Here's how the part is built. I have some questions about the finished solid (model axes, mm). Face numbers are marked on the shaded views. A direction names the side the tool comes from. Coordinates: 2 decimals unless noted, no trailing zeros. Write each loop counter-clockwise with the first axis right and the second up, starting at its lowest first coordinate (ties: lowest second). Pieces come first, ordered by that corner, then holes. Notation, with made-up numbers: (61, 14.5) - (118, 14.5) arc R27 ccw to (118, 50.5) - close; hole circle Ø8 at (-5, -39). An arc over 180 degrees is marked (long way). Answer in a Markdown table with one row per item. Add a question column.
Item 1: Which directions (+Z, -Z, +X, -X, +Y, -Y) give clear straight access to the entire face, cutting with the end or side of a thin tool? Please do the marked faces 1 and 2.
Item 2: Imagine slicing it at C-C (x = -13). Please give me the cut outline in (y, z), plus the area to 3 significant figures.
Item 3: I'm going to push a flat-ended pin straight in: pin 1 (10 mm diameter, centred on x = 4, y = -33, fed in from -Z). Where does the tip first touch, or does it pass through?
Item 4: If I drill on probe 1 along X at (y, z) = (-14.5, 38); probe 2 along Z at (x, y) = (-0.5, -12), over which ranges is the centre line in solid material (lowest first)? Write a range as from..to.
Item 5: Imagine slicing it at B-B (y = 33). Please give me the cut outline in (x, z).
Item 6: Imagine slicing it at A-A (z = 20.5). Please give me the cut outline in (x, y).
Item 7: We'd pull the mould along X, two halves only. Please class the marked faces 3, 4 and 5: +X half, -X half, draft (parallel to the pull), parting line (faces both ways), or undercut.
from build123d import *

# Parameters (mm, degrees)
F0_W     = 100
F0_H     = 100
F1_DEPTH = 100
F2_W     = 100
F2_H     = 64.8081071675
F3_DEPTH = 40
F4_W     = 60
F4_H     = 40
F5_DEPTH = 100.001
F6_DEPTH = 40


with BuildPart() as f1:
    # F0 (on Top) → F1 (new body)
    with BuildSketch(Plane.XY):
        Rectangle(F0_W, F0_H)
    extrude(amount=F1_DEPTH)

    # F2 (on face) → F3 (cut)
    with BuildSketch(Plane.XY.offset(100)):
        with Locations((0, -17.5959464163)):
            Rectangle(F2_W, F2_H)
    extrude(amount=-F3_DEPTH, mode=Mode.SUBTRACT)

    # F4 (on face) → F5 (cut, through all)
    with BuildSketch(Plane.XZ.offset(50)):
        with Locations((0, 20)):
            Rectangle(F4_W, F4_H)
    extrude(amount=-F5_DEPTH, mode=Mode.SUBTRACT)

    # F6 (add): a face of the model
    f6_faces = [f1.faces().sort_by_distance(p)[0] for p in [
        (0, -17.5959464163, 60),
    ]]
    extrude(f6_faces, amount=F6_DEPTH)


solid = f1.part
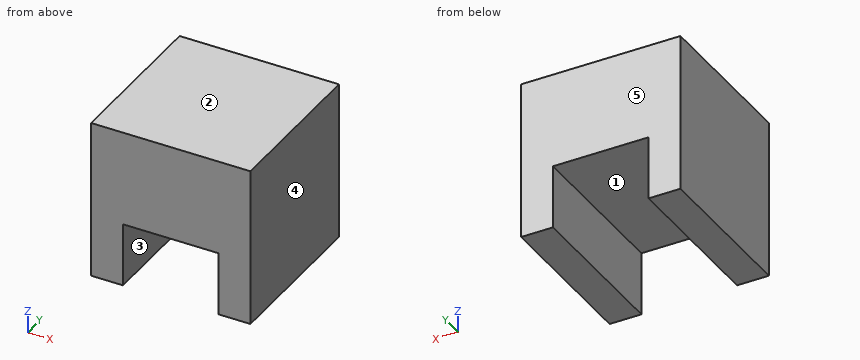
Here are the results:
| question | item | result |
|---|---|---|
| 1 | face 1 | -Z, +Y, -Y |
| 1 | face 2 | +Z, +X, -X, +Y, -Y |
| 2 | outline | (-50, 40) - (50, 40) - (50, 100) - (-50, 100) - close |
| 2 | area | 6,000 mm2 |
| 3 | pin 1 | stops at z = 40 |
| 4 | probe 1 | x = -50..-30, 30..50 |
| 4 | probe 2 | z = 40..100 |
| 5 | outline | (-50, 0) - (-30, 0) - (-30, 40) - (30, 40) - (30, 0) - (50, 0) - (50, 100) - (-50, 100) - close |
| 6 | outline | (-50, -50) - (-30, -50) - (-30, 50) - (-50, 50) - close; (30, -50) - (50, -50) - (50, 50) - (30, 50) - close |
| 7 | face 3 | undercut |
| 7 | face 4 | +X half |
| 7 | face 5 | draft |
